```python
from build123d import *

# Parameters (mm, degrees)
F0_W     = 412.447963
F0_H     = 8.529411
F0_H_2   = 8.529412
F1_DEPTH = 3


# Not quite as in the source:
# - ends of sketch curves that miss each other by under 0.0002 mm in the source are joined


with BuildPart() as f1:
    # F0 (on Front) → F1 (new body)
    with BuildSketch(Plane.XZ):
        with BuildLine():
            Line((-245, 131.615385), (-245, -131.615384))
            ThreePointArc((-245, -131.615384), (-241.0797377372, -141.0797367372), (-231.615385, -145))
            Line((-231.615385, -145), (231.615384, -145))
            ThreePointArc((231.615384, -145), (241.0797367372, -141.0797367372), (245, -131.615384))
            Line((245, -131.615384), (245, 131.615385))
            ThreePointArc((245, 131.615385), (241.0797367372, 141.0797377372), (231.615384, 145.000001))
            Line((231.615384, 145.000001), (-231.615385, 145))
            ThreePointArc((-231.615385, 145), (-241.0797377372, 141.0797377372), (-245, 131.615385))
        make_face()
        with BuildLine():
            ThreePointArc((-223.67647, -115.147058), (-221.1782633576, -121.1782623576), (-215.147059, -123.676469))
            Line((-215.147059, -123.676469), (-215.147059, -132.205882))
            Line((-215.147059, -132.205882), (-219.411765, -132.205882))
            ThreePointArc((-219.411765, -132.205882), (-228.4585725971, -128.4585725971), (-232.205883, -119.411765))
            Line((-232.205883, -119.411765), (-232.205883, 119.411764))
            ThreePointArc((-232.205883, 119.411764), (-228.4585725971, 128.4585715971), (-219.411765, 132.205882))
            Line((-219.411765, 132.205882), (-215.147059, 132.205883))
            Line((-215.147059, 132.205883), (-215.147059, 123.676471))
            ThreePointArc((-215.147059, 123.676471), (-221.1782633576, 121.1782633576), (-223.67647, 115.147059))
            Line((-223.67647, 115.147059), (-223.67647, -115.147058))
        make_face(mode=Mode.SUBTRACT)
        with BuildLine():
            ThreePointArc((-70.7599172527, 5.5663826998), (-137.2958198093, -88.6390266704), (-87.6127799718, 15.4440220749))
            Line((-87.6127799718, 15.4440220749), (-91.766694, 1.50065))
            ThreePointArc((-91.766694, 1.50065), (-133.2066284732, -74.0292729296), (-75.3272882753, -10.2168972398))
            Line((-75.3272882753, -10.2168972398), (-70.7599172527, 5.5663826998))
        make_face(mode=Mode.SUBTRACT)
        with BuildLine():
            Line((-68.723593, 12.582627), (-64.743288, 26.326147))
            Line((-64.743288, 26.326147), (3.159571, -20.475886))
            ThreePointArc((3.159571, -20.475886), (3.3683994767, -20.3043898267), (3.5792137936, -20.1353407395))
            Line((3.5792137936, -20.1353407395), (7.411744, -26.95528))
            ThreePointArc((7.411744, -26.95528), (4.0249471652, -31.5409295129), (2.5258681402, -37.0410509302))
            Line((2.5258681402, -37.0410509302), (-68.723593, 12.582627))
        make_face(mode=Mode.SUBTRACT)
        with Locations((-5e-07, -127.9411765)):
            Rectangle(F0_W, F0_H, mode=Mode.SUBTRACT)
        with BuildLine():
            Line((22.72508, -68.805566), (30.090636, -68.805566))
            Line((30.090636, -68.805566), (21.674726, -53.339399))
            ThreePointArc((21.674726, -53.339399), (24.591046355, -52.3025256725), (27.243072314, -50.7066594202))
            Line((27.243072314, -50.7066594202), (36.565765, -68.805566))
            Line((36.565765, -68.805566), (45.281341, -68.805566))
            Line((45.281341, -68.805566), (45.281341, -76.614964))
            Line((45.281341, -76.614964), (22.72508, -76.614964))
            Line((22.72508, -76.614964), (22.72508, -68.805566))
        make_face(mode=Mode.SUBTRACT)
        with BuildLine():
            Line((-4.847605, -34.261624), (2.51358, -39.388528))
            ThreePointArc((2.51358, -39.388528), (8.0448119147, -50.1939653909), (19.6676101132, -53.6957600257))
            Line((19.6676101132, -53.6957600257), (23.527377, -60.788967))
            ThreePointArc((23.527377, -60.788967), (2.1451797481, -55.2211156409), (-4.847605, -34.261624))
        make_face(mode=Mode.SUBTRACT)
        with BuildLine():
            ThreePointArc((83.96580189, 15.3881272867), (154.3064474066, -68.0805916135), (47.3881182197, -46.096407971))
            Line((47.3881182197, -46.096407971), (62.056469, -46.096408))
            ThreePointArc((62.056469, -46.096408), (141.8170821306, -60.7137946065), (91.0686279767, 2.5318990705))
            Line((91.0686279767, 2.5318990705), (83.96580189, 15.3881272867))
        make_face(mode=Mode.SUBTRACT)
        with BuildLine():
            Line((8.930442, -25.711427), (-1.213114, -7.6611))
            Line((-1.213114, -7.6611), (-9.807377, -7.6611))
            Line((-9.807377, -7.6611), (-9.807377, 0.1483))
            Line((-9.807377, 0.1483), (12.748884, 0.1483))
            Line((12.748884, 0.1483), (12.748884, -7.6611))
            Line((12.748884, -7.6611), (5.767885, -7.6611))
            Line((5.767885, -7.6611), (14.045243, -23.30707))
            ThreePointArc((14.045243, -23.30707), (11.3772825006, -24.2740536292), (8.930442, -25.711427))
        make_face(mode=Mode.SUBTRACT)
        with BuildLine():
            ThreePointArc((47.3586275037, -31.2217609366), (54.5791913728, -9.7531888086), (69.4990666913, 7.2889194025))
            Line((69.4990666913, 7.2889194025), (76.442916, -5.74499))
            ThreePointArc((76.442916, -5.74499), (67.0095000702, -17.2261004781), (62.0168330844, -31.2217610145))
            Line((62.0168330844, -31.2217610145), (47.3586275037, -31.2217609366))
        make_face(mode=Mode.SUBTRACT)
        with BuildLine():
            Line((90.984376, -29.244421), (57.508949, 33.590423))
            Line((57.508949, 33.590423), (63.619612, 48.524677))
            Line((63.619612, 48.524677), (110.016211, -35.453915))
            ThreePointArc((110.016211, -35.453915), (109.9324845309, -41.3751059281), (104.790172, -44.311794))
            Line((104.790172, -44.311794), (40.343874, -44.311793))
            ThreePointArc((40.343874, -44.311793), (37.3331086152, -51.0181961304), (32.3730594707, -56.443918593))
            Line((32.3730594707, -56.443918593), (28.754286, -49.418498))
            ThreePointArc((28.754286, -49.418498), (33.3103193803, -40.4589080248), (31.409337593, -30.5888542334))
            Line((31.409337593, -30.5888542334), (34.77995, -22.351191))
            ThreePointArc((34.77995, -22.351191), (38.3615541693, -27.2968191094), (40.5267526716, -33.006376077))
            Line((40.5267526716, -33.006376077), (88.726046, -33.006377))
            ThreePointArc((88.726046, -33.006377), (90.9199219225, -31.7645528859), (90.984376, -29.244421))
        make_face(mode=Mode.SUBTRACT)
        with BuildLine():
            Line((219.411764, -132.205882), (215.147059, -132.205882))
            Line((215.147059, -132.205882), (215.147059, -123.676471))
            ThreePointArc((215.147059, -123.676471), (221.1782633576, -121.1782623576), (223.67647, -115.147058))
            Line((223.67647, -115.147058), (223.67647, 115.147059))
            ThreePointArc((223.67647, 115.147059), (221.1782633576, 121.1782633576), (215.147059, 123.67647))
            Line((215.147059, 123.67647), (215.147059, 132.205883))
            Line((215.147059, 132.205883), (219.411764, 132.205882))
            ThreePointArc((219.411764, 132.205882), (228.4585715971, 128.4585715971), (232.205882, 119.411764))
            Line((232.205882, 119.411764), (232.205881, -119.411765))
            ThreePointArc((232.205881, -119.411765), (228.4585715971, -128.4585725971), (219.411764, -132.205882))
        make_face(mode=Mode.SUBTRACT)
        with BuildLine():
            ThreePointArc((-72.4661841519, 65.5207366103), (-82.1538966479, 83.216021136), (-66.4060260229, 95.8247260113))
            Line((-66.4060260229, 95.8247260113), (-40.035993, 95.824726))
            Line((-40.035993, 95.824726), (-40.035993, 80.630917))
            Line((-40.035993, 80.630917), (-64.424786, 80.630917))
            ThreePointArc((-64.424786, 80.630917), (-66.0282591874, 79.5071913113), (-65.5192035969, 77.616491482))
            Line((-65.5192035969, 77.616491482), (-59.43939, 72.531557))
            ThreePointArc((-59.43939, 72.531557), (-56.3975970197, 66.4763179948), (-56.9296708586, 59.7209263141))
            Line((-56.9296708586, 59.7209263141), (-77.850161, -12.515038))
            ThreePointArc((-77.850161, -12.515038), (-87.3559409811, -31.7459411903), (-105.0135430166, -43.9277549547))
            ThreePointArc((-105.0135430166, -43.9277549547), (-112.4545221205, -41.478665578), (-111.0494858176, -33.7720412284))
            ThreePointArc((-111.0494858176, -33.7720412284), (-101.1018664771, -25.9057272999), (-94.7919815143, -14.9048461665))
            Line((-94.7919815143, -14.9048461665), (-71.450754, 63.444245))
            ThreePointArc((-71.450754, 63.444245), (-71.5531660844, 64.6806886283), (-72.4661841519, 65.5207366103))
        make_face(mode=Mode.SUBTRACT)
        Polygon((-61.428563, 37.771498), (-57.350449, 51.85274), (44.398561, 51.85274), (38.504827, 37.771498), align=None, mode=Mode.SUBTRACT)
        with BuildLine():
            ThreePointArc((12.2794031528, -15.8349486032), (15.2656197234, -15.2838363253), (18.2982629962, -15.1279872662))
            Line((18.2982629962, -15.1279872662), (51.823582, 64.970319))
            ThreePointArc((51.823582, 64.970319), (51.7665690353, 66.512857989), (50.4881340177, 67.3778901407))
            ThreePointArc((50.4881340177, 67.3778901407), (39.4345578147, 69.3755880777), (28.6570272111, 72.5405805985))
            ThreePointArc((28.6570272111, 72.5405805985), (26.2908771018, 75.8079169957), (27.8157723755, 79.5427327786))
            ThreePointArc((27.8157723755, 79.5427327786), (28.3174115009, 79.8213352122), (28.883051, 79.917843))
            Line((28.883051, 79.917843), (83.068308, 79.917844))
            ThreePointArc((83.068308, 79.917844), (83.7102572475, 79.6265153128), (83.9136824011, 78.9515420803))
            ThreePointArc((83.9136824011, 78.9515420803), (79.0432795601, 69.2443269594), (69.2278859862, 64.5957881246))
            ThreePointArc((69.2278859862, 64.5957881246), (68.3724892885, 64.249714451), (67.8224577861, 63.5088130817))
            Line((67.8224577861, 63.5088130817), (30.106815, -28.666942))
            ThreePointArc((30.106815, -28.666942), (23.8211455462, -23.950033286), (16.0297460076, -22.92389506))
            Line((16.0297460076, -22.92389506), (12.2794031528, -15.8349486032))
        make_face(mode=Mode.SUBTRACT)
        with Locations((-5e-07, 127.941177)):
            Rectangle(F0_W, F0_H_2, mode=Mode.SUBTRACT)
    extrude(amount=F1_DEPTH)


solid = f1.part
```
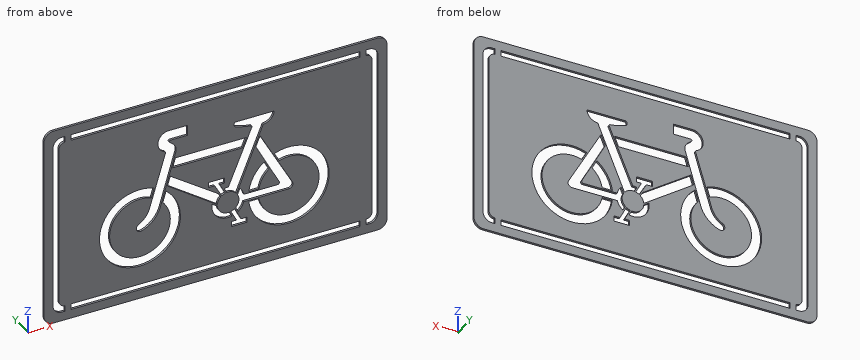
Model file for the job. Use its own axes, mm. Round coordinates to 2 decimals unless told otherwise and drop trailing zeros. Order: outer loops, then holes, each group sorted by start corner. A loop starts at its lowest first (then second) coordinate and runs counter-clockwise, first axis right, second up. Notation, with made-up numbers: M -19,61.5 L -7,61.5 A5 cw -7,65.5 Z; hole C 64,23 d11. An arc over 180 degrees is marked long. Use CSV: the item, a comma, the result in double quotes.
Item 1: Saw through at A-A (x = -200). List the corners of the cut face in (y, z), plus the area to 3 significant figures.
Worked answers:
outline,"M -3,-145 L 0,-145 L 0,-132.21 L -3,-132.21 Z; M -3,-123.68 L 0,-123.68 L 0,123.68 L -3,123.68 Z; M -3,132.21 L 0,132.21 L 0,145 L -3,145 Z"
area,"819 mm²"
Item 2: Probe probe 1 along X at (y, z) = (-1.3, -107.5); probe 2 along Z at (x, y) = (171, -1.2); probe 3 along Z at (x, y) = (100, -0.85). List the from-to ranges inside material, lowest first.
Worked answers:
probe 1,"-245 to -232.21, -223.68 to 223.68, 232.21 to 245"
probe 2,"-145 to -132.21, -123.68 to 123.68, 132.21 to 145"
probe 3,"-145 to -132.21, -123.68 to -96.12, -81.56 to -44.31, -17.32 to 4.47, 19.03 to 123.68, 132.21 to 145"
Item 3: Saw through at B-B (x = 133.5). List the corners of the cut face in (y, z), plus the area to 3 significant figures.
Worked answers:
outline,"M -3,-145 L 0,-145 L 0,-132.21 L -3,-132.21 Z; M -3,-123.68 L 0,-123.68 L 0,-88.6 L -3,-88.6 Z; M -3,-70.8 L 0,-70.8 L 0,-6.29 L -3,-6.29 Z; M -3,11.51 L 0,11.51 L 0,123.68 L -3,123.68 Z; M -3,132.21 L 0,132.21 L 0,145 L -3,145 Z"
area,"712 mm²"
Item 4: Saw through at C-C (y = -2.5). State how many separate pieces and enclosed holes the cut face has, plus the area to 3 significant figures.
Worked answers:
separate pieces,"1"
enclosed holes,"15"
area,"111,000 mm²"
